```python
from build123d import *

# Parameters (mm, degrees)
F1_DEPTH  = 155.575
F2_R      = 3.69316
F3_R      = 1.98374
F7_DEPTH  = 155.575
F8_R      = 2.5
F9_DEPTH  = 162.96132
F10_R     = 5.674995
F11_R     = 1.35255
F12_DEPTH = 1.70942
F13_W     = 3.69316
F13_H     = 75.7569519651
F14_DEPTH = 3.69316


with BuildPart() as f1:
    # F0 (on Top) → F1 (new body)
    with BuildSketch(Plane.XY):
        Polygon((0, 0), (-1.70942, 0), (-1.70942, -18.8265943), (161.2519, -18.8265943), (161.2519, 0), (159.54248, 0), (159.54248, -17.1171743), (0, -17.1171743), align=None)
    extrude(amount=F1_DEPTH)

    # F2
    f2_edges = [f1.edges().sort_by_distance(p)[0] for p in [
        (161.2519, -18.826594, 77.7875),
        (-1.70942, -18.826594, 77.7875),
    ]]
    fillet(f2_edges, radius=F2_R)

    # F3
    f3_edges = [f1.edges().sort_by_distance(p)[0] for p in [
        (159.54248, -17.117174, 77.7875),
        (0, -17.117174, 77.7875),
    ]]
    fillet(f3_edges, radius=F3_R)

    # F5 (on offset) → F7 (join, through all)
    with BuildSketch(Plane.YZ.offset(1.98374)):
        with BuildLine():
            Line((-17.1171743, 0), (-18.8265943, 0))
            ThreePointArc((-18.8265943, 0), (-17.74489278, -2.61145848), (-15.1334343, -3.69316))
            Line((-15.1334343, -3.69316), (0, -3.69316))
            Line((0, -3.69316), (0, -1.98374))
            Line((0, -1.98374), (-15.1334343, -1.98374))
            ThreePointArc((-15.1334343, -1.98374), (-16.5361503061, -1.4027160061), (-17.1171743, 0))
        make_face()
    extrude(amount=F7_DEPTH)

    # F8 (on face) → F9 (cut, through all)
    with BuildSketch(Plane(origin=(-1.70942, 0, 0), x_dir=(0, -1, 0), z_dir=(-1, 0, 0))):
        with Locations((5.675, 149.9)):
            Circle(F8_R)
        with Locations((5.675, 86.8541635573)):
            Circle(F8_R)
        with BuildLine():
            ThreePointArc((2.8375, 81.9394693908), (0.7603058335, 84.0166635573), (0, 86.8541635573))
            Line((0, 86.8541635573), (0, 0))
            Line((0, 0), (15.1334343, 0))
            Line((15.1334343, 0), (15.1334343, 75.7569519651))
            Line((15.1334343, 75.7569519651), (13.5459343, 75.7569519651))
            Line((13.5459343, 75.7569519651), (2.8375, 81.9394693908))
        make_face()
    extrude(amount=-F9_DEPTH, mode=Mode.SUBTRACT)

    # F10
    f10_edges = [f1.edges().sort_by_distance(p)[0] for p in [
        (-0.85471, 0, 155.575),
        (160.39719, 0, 155.575),
    ]]
    fillet(f10_edges, radius=F10_R)

    # F11 (on face) → F12 (cut, through all)
    with BuildSketch(Plane(origin=(0, -17.1171743, 0), x_dir=(-1, 0, 0), z_dir=(0, 1, 0))):
        with Locations((-25.8627459407, 59.7118170977)):
            Circle(F11_R)
        with Locations((-25.8627459407, 105.6590335488)):
            Circle(F11_R)
        with Locations((-25.8627459407, 151.60625)):
            Circle(F11_R)
        with Locations((-133.6797340593, 151.60625)):
            Circle(F11_R)
        with Locations((-133.6797340593, 105.6590335488)):
            Circle(F11_R)
        with Locations((-133.6797340593, 59.7118170977)):
            Circle(F11_R)
    extrude(amount=-F12_DEPTH, mode=Mode.SUBTRACT)

    # F13 (on face) → F14 (cut, through all)
    with BuildSketch(Plane.XZ.offset(18.8265943)):
        with Locations((0.13716, 37.8784759826)):
            Rectangle(F13_W, F13_H)
        with Locations((159.40532, 37.8784759826)):
            Rectangle(F13_W, F13_H)
    extrude(amount=-F14_DEPTH, mode=Mode.SUBTRACT)


solid = f1.part
```
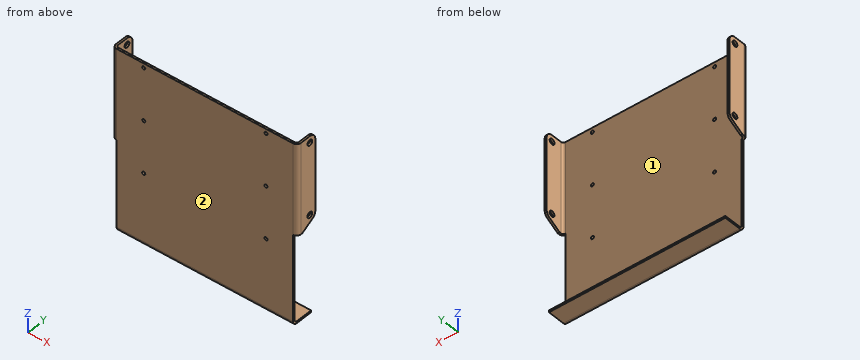
Here's how the part is built. I have some questions about the finished solid (model axes, mm). Face numbers are marked on the shaded views. Round coordinates to 2 decimals unless told otherwise and drop trailing zeros. Order: outer loops, then holes, each group sorted by start corner. A loop starts at its lowest first (then second) coordinate and runs counter-clockwise, first axis right, second up. Notation, with made-up numbers: (-8, 39.5) -> (50, 39.5) arc R19 ccw to (50, 63.5) -> close; hole circle Ø9 at (-3, -22.5). An arc over 180 degrees is marked (long way). Use a Markdown table: item, result. Add a question column.
(1) I need wall thicknesses on line 1 along X through (y, z) = (-5.25, 93); line 2 along Y through (x, z) = (133.5, 117.5); line 3 along Z through (x, y) = (136, -17.5) (3 decimals). Which ranges of each line are inside material? Lowest first, please.
(2) Suppose I cut it at A-A, the plane x = 14.5. Please give me the cut outline in (y, z) (3 decimals).
(3) Suppose I cut it at B-B, the plane z = 125.5. Please give me the cut outline in (x, y), and give its area (3 significant figures).
(4) Suppose I cut it at D-D, the plane z = 36. Please give me the cut outline in (x, y), and give its area (3 significant figures).
(5) Suppose I cut it at C-C, the plane y = -10.5. Please give me the cut outline in (x, z) (3 decimals), and give its area (3 significant figures).
(6) If we mould it in two halves opening along X, with no side actions, what happens to the marked faces 1 and 2? For each: released by +X, released by -X, zero draft, split by the parting line, or undercut.
(7) For pin 1 Ø9.5 at (y, z) = (-8, 55.5) entering from +X; pin 2 Ø4.5 at (x, y) = (56.5, -6.5) entering from +Z; pin 3 Ø3 at (x, z) = (114, 138) entering from +Y; pin 4 Ø1.1 at (x, y) = (160, -15) entering from -Z, each with a flat end and sliding along its axis, tell me the tip position at first contact or that it passes through.
Verdict:
| question | item | result |
|---|---|---|
| 1 | line 1 | -1.71 to 0, 159.54 to 161.25 |
| 1 | line 2 | -18.83 to -17.12 |
| 1 | line 3 | -2.835 to 155.575 |
| 2 | outline | (-18.827, 0) arc R3.693 ccw to (-15.133, -3.693) -> (0, -3.693) -> (0, -1.984) -> (-15.133, -1.984) arc R1.984 cw to (-17.117, 0) -> (-17.117, 155.575) -> (-18.827, 155.575) -> close |
| 3 | outline | (-1.71, -15.13) arc R3.69 ccw to (1.98, -18.83) -> (157.56, -18.83) arc R3.69 ccw to (161.25, -15.13) -> (161.25, 0) -> (159.54, 0) -> (159.54, -15.13) arc R1.98 cw to (157.56, -17.12) -> (1.98, -17.12) arc R1.98 cw to (0, -15.13) -> (0, 0) -> (-1.71, 0) -> close |
| 3 | area | 333 mm2 |
| 4 | outline | (1.98, -18.83) -> (157.56, -18.83) -> (157.56, -17.12) -> (1.98, -17.12) -> close |
| 4 | area | 266 mm2 |
| 5 | outline | (-1.709, 77.516) -> (0, 77.516) -> (0, 155.575) -> (-1.709, 155.575) -> close; (1.984, -3.693) -> (157.559, -3.693) -> (157.559, -1.984) -> (1.984, -1.984) -> close; (159.542, 77.516) -> (161.252, 77.516) -> (161.252, 155.575) -> (159.542, 155.575) -> close |
| 5 | area | 533 mm2 |
| 6 | face 1 | undercut |
| 6 | face 2 | zero draft |
| 7 | pin 1 | through |
| 7 | pin 2 | z = -1.98 |
| 7 | pin 3 | y = -17.12 |
| 7 | pin 4 | z = 75.76 |
